Can you work these out from the drawing? Everything is in mm from the part's minimum corner. Round coordinates to 2 decimals unless told otherwise and drop trailing zeros. Loops run counter-clockwise (first coordinate to the right, second up) from the corner with the lowest first, then second, coordinate; pieces in that order, holes last. Notation, with made-up numbers: M 34.5,59.5 L 65.5,59.5 A14 ccw 65.5,65.5 Z; hole C 89.5,62 d11. An arc over 180 degrees is marked long. Use a Markdown table: item, result.
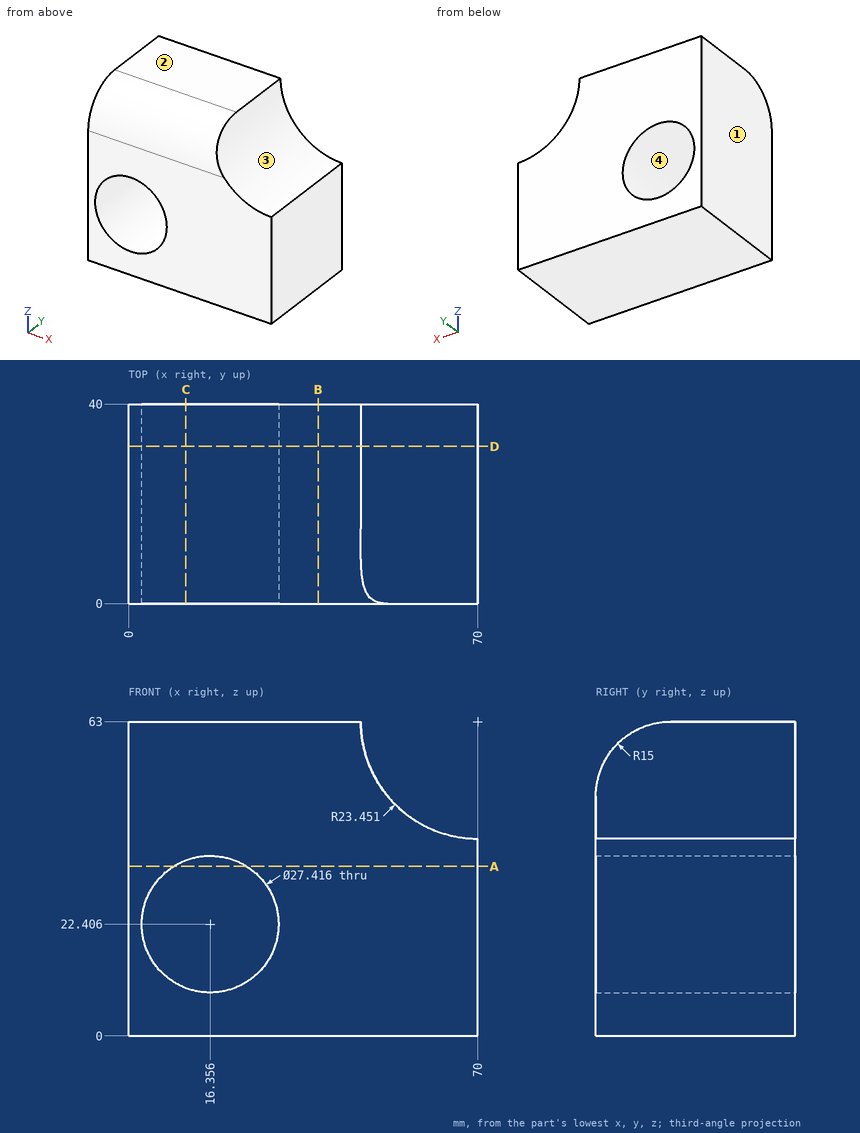
Q1. Imagine slicing it at C-C, the plane x = 11.5. Please give me the cut outline in (y, z) (1 decimal), then the cut area to 3 significant figures.
Return value:
| item | result |
|---|---|
| outline | M 0,0 L 40,0 L 40,9.6 L 0,9.6 Z; M 0,35.2 L 40,35.2 L 40,63 L 15,63 A15 ccw 0,48 Z |
| area | 1,450 mm^2 |
Q2. I need wall thicknesses on line 1 (Z direction, x = 13, y = 14.5) (1 decimal); line 2 (X direction, y = 9, z = 15); line 3 (Z direction, x = 4, y = 38.5) (1 decimal). Which ranges of each line are inside material? Lowest first, please. Write a range as from..to.
Return value:
| item | result |
|---|---|
| line 1 | z = 0..9.1, 35.7..63 |
| line 2 | x = 0..4.82, 27.89..70 |
| line 3 | z = 0..16.5, 28.3..63 |
Q3. We'd pull the mould along X, two halves only. Please class the marked faces 1, 2, 3 and 4: pulls with the +X half, pulls with the -X half, needs draft (parallel to the pull), parting line crosses it, or undercut.
Return value:
| item | result |
|---|---|
| face 1 | pulls with the -X half |
| face 2 | needs draft |
| face 3 | pulls with the +X half |
| face 4 | undercut |
Q4. Will these pins go through, and if not, where does the flat tip stop? P1, Ø1.5, axis at x = 28, y = 5, coming from the +Z side; P2, Ø6, axis at x = 62.5, y = 15, coming from the +Z side.
Return value:
| item | result |
|---|---|
| P1 | stops at z = 59.81 |
| P2 | stops at z = 42.03 |
Q5. Imagine slicing it at A-A, the plane z = 34. Please give me the cut outline in (x, y), then the cut area to 4 significant figures.
Return value:
| item | result |
|---|---|
| outline | M 0,0 L 9.04,0 L 9.04,40 L 0,40 Z; M 23.67,0 L 70,0 L 70,40 L 23.67,40 Z |
| area | 2,215 mm^2 |
Q6. Imagine slicing it at B-B, the plane x = 38. Please give me the cut outline in (y, z).
Return value:
| item | result |
|---|---|
| outline | M 0,0 L 40,0 L 40,63 L 15,63 A15 ccw 0,48 Z |
Q7. Imagine slicing it at D-D, the plane y = 31.5. Please give me the cut outline in (x, z) (1 decimal), then the cut area to 3 significant figures.
Return value:
| item | result |
|---|---|
| outline | M 0,0 L 70,0 L 70,39.5 A23.5 cw 46.5,63 L 0,63 Z; hole C 16.4,22.4 d27.4 |
| area | 3,390 mm^2 |
